For this review, take the finished solid that the model builds, in its own axes (mm). Face numbers are marked on the shaded views. A direction names the side the tool comes from. Round coordinates to 2 decimals unless told otherwise and drop trailing zeros. Order: outer loops, then holes, each group sorted by start corner. A loop starts at its lowest first (then second) coordinate and runs counter-clockwise, first axis right, second up.
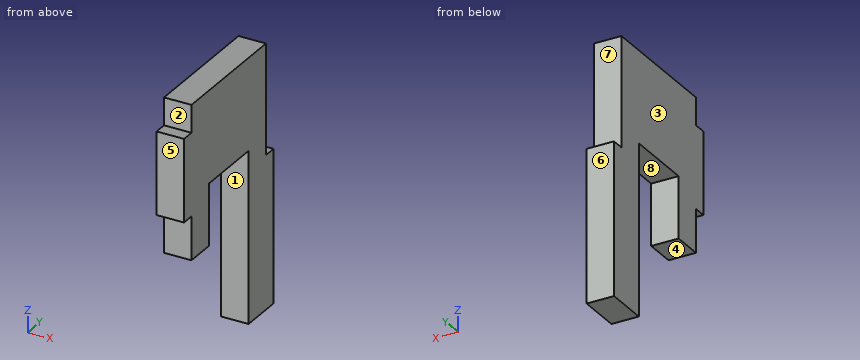
```python
from build123d import *

# Parameters (mm, degrees)
SKETCH1_W           = 16.5
SKETCH1_H           = 43
BOSS_EXTRUDE1_DEPTH = 3.175
SKETCH2_W           = 9.525
SKETCH2_H           = 1.5
CUT_EXTRUDE1_DEPTH  = 10
SKETCH3_W           = 28.475
SKETCH3_H           = 11.5
CUT_EXTRUDE2_DEPTH  = 4.175
SKETCH5_W           = 3.175
SKETCH5_H           = 15
BOSS_EXTRUDE2_DEPTH = 3.175
SKETCH6_W           = 15.854218726
SKETCH6_H           = 5
SKETCH6_W_2         = 7.106349473
SKETCH6_H_2         = 8.006430413
CUT_EXTRUDE4_DEPTH  = 10
SKETCH7_W           = 9.525
SKETCH7_H           = 1.5
BOSS_EXTRUDE3_DEPTH = 3.175


with BuildPart() as part:
    # Sketch1 → Boss-Extrude1 (new body)
    with BuildSketch(Plane(origin=(0, 0, 0), x_dir=(0, -1, 0), z_dir=(1, 0, 0))):
        with Locations((8.25, 21.5)):
            Rectangle(SKETCH1_W, SKETCH1_H)
    extrude(amount=BOSS_EXTRUDE1_DEPTH)

    # Sketch2 → Cut-Extrude1 (cut)
    with BuildSketch(Plane(origin=(3.175, 0, 0), x_dir=(0, 0, -1), z_dir=(1, 0, 0))):
        with Locations((4.7625, -0.75)):
            Rectangle(SKETCH2_W, SKETCH2_H)
    extrude(amount=-CUT_EXTRUDE1_DEPTH, mode=Mode.SUBTRACT)

    # Sketch3 → Cut-Extrude2 (cut, through all)
    with BuildSketch(Plane(origin=(3.175, 0, 0), x_dir=(0, 0, -1), z_dir=(1, 0, 0))):
        with Locations((28.7625, -10.75)):
            Rectangle(SKETCH3_W, SKETCH3_H)
    extrude(amount=-CUT_EXTRUDE2_DEPTH, mode=Mode.SUBTRACT)

    # Sketch5 → Boss-Extrude2 (add)
    with BuildSketch(Plane(origin=(3.175, 0, 0), x_dir=(0, 0, -1), z_dir=(1, 0, 0))):
        with Locations((-1.5875, -9)):
            Rectangle(SKETCH5_W, SKETCH5_H)
    extrude(amount=-BOSS_EXTRUDE2_DEPTH)

    # Sketch6 → Cut-Extrude4 (cut)
    with BuildSketch(Plane(origin=(3.175, 0, 0), x_dir=(0, 0, -1), z_dir=(1, 0, 0))):
        with Locations((35.072890637, -2.5)):
            Rectangle(SKETCH6_W, SKETCH6_H)
        with Locations((10.971825264, -9.003215207)):
            Rectangle(SKETCH6_W_2, SKETCH6_H_2)
    extrude(amount=-CUT_EXTRUDE4_DEPTH, mode=Mode.SUBTRACT)

    # Sketch7 → Boss-Extrude3 (add)
    with BuildSketch(Plane(origin=(3.175, 0, 0), x_dir=(0, 0, -1), z_dir=(1, 0, 0))):
        with Locations((4.7625, -17.25)):
            Rectangle(SKETCH7_W, SKETCH7_H)
    extrude(amount=-BOSS_EXTRUDE3_DEPTH)


solid = part.part
```
Q1. Take a section at D-D, the plane z = -0.5. State the section outline as (x, y) points (3 decimals).
Q2. Take a section at A-A, the plane z = -11. State the section outline as (x, y) points (3 decimals), plus the area to 3 significant figures.
Q3. Mouldability with a two-part tool opening along Y and no side actions: class the marked faces 1, 2 and 3 as +Y half, -Y half, draft (parallel to the pull), parting line (faces both ways), or undercut.
Q4. Tool access review of the marked faces 4, 5, 6, 7 and 8: name each direction out of +Z, -Z, +X, -X, +Y, -Y from which nothing blocks a thin tool from reaching the whole face with its end or side.
Q5. Wall thickness on line 1 (Y direction, x = 0.8, z = -13.5); line 2 (Y direction, x = 2.55, z = -8); line 3 (Z direction, x = 0.15, y = -12) (3 decimals): over which ranges is each line inside the solid? List them lowest first.
Q6. Take a section at B-B, the plane x = 0.65. State the section outline as (y, z) points (3 decimals).
Q7. Take a section at C-C, the plane y = -11.25. State the section outline as (x, z) points (3 decimals), plus the area to 3 significant figures.
Q8. Clearance check with flat-ended pins moving along their axes: pin 1 (0.8 mm diameter, centred on x = 2, y = -17.5, fed in from +Z); pin 2 (3 mm diameter, centred on y = -7.5, z = -14, fed in from +X). State where each tip first meets the part, or that it passes through.
Working result:
1. outline: (0, -18) - (3.175, -18) - (3.175, -1.5) - (0, -1.5) - close
2. outline: (0, -16.5) - (3.175, -16.5) - (3.175, -13.006) - (0, -13.006) - close; (0, -5) - (3.175, -5) - (3.175, 0) - (0, 0) - close
2. area: 27.0 mm2
3. face 1: undercut
3. face 2: -Y half
3. face 3: draft
4. face 4: -Z, +X, -X, -Y
4. face 5: +Z, -Z, +X, -X, -Y
4. face 6: +Z, -Z, +X, -X, +Y
4. face 7: +Z, +X, -X, +Y
4. face 8: -Z, +X, -X
5. line 1: y = -16.5 to -13.01, -5 to 0
5. line 2: y = -18 to -13.01, -5 to -1.5
5. line 3: z = -7.419 to 3.175
6. outline: (-18, -9.525) - (-16.5, -9.525) - (-16.5, -14.525) - (-13.006, -14.525) - (-13.006, -7.419) - (-5, -7.419) - (-5, -27.146) - (0, -27.146) - (0, -9.525) - (-1.5, -9.525) - (-1.5, 3.175) - (-16.5, 3.175) - (-16.5, 0) - (-18, 0) - close
7. outline: (0, -7.419) - (3.175, -7.419) - (3.175, 3.175) - (0, 3.175) - close
7. area: 33.6 mm2
8. pin 1: stops at z = 0
8. pin 2: passes through
